Here's how the part is built. I have some questions about the finished solid (model axes, mm). Face numbers are marked on the shaded views. A direction names the side the tool comes from. Round coordinates to 2 decimals unless told otherwise and drop trailing zeros. Write each loop counter-clockwise with the first axis right and the second up, starting at its lowest first coordinate (ties: lowest second). Pieces come first, ordered by that corner, then holes. Notation, with made-up numbers: (82, 62) - (108, 62) arc R11 ccw to (108, 80) - close; hole circle Ø9 at (2.5, 53). An arc over 180 degrees is marked (long way). One line per question, with ' | ' between items. Start each with the question number.
(1) Imagine slicing it at A-A (y = 0). Write out the boundary of the cut face in (x, z), plus the area to 3 significant figures.
(2) Will these pins go through, and if not, where does the flat tip stop? pin 1 (4 mm diameter, centred on y = 8, z = 7.5, fed in from -X); pin 2 (12 mm diameter, centred on x = -42, y = 27.5, fed in from +Z); pin 3 (1 mm diameter, centred on y = -12.5, z = 2.5, fed in from +X).
(3) Thinking about a two-plate mould opening in X: for the marked faces 3, 4 and 5, which applies, pulls with the +X half, pulls with the -X half, needs draft (parallel to the pull), parting line crosses it, or undercut?
(4) For the marked faces 1 and 2, which set-ups out of +Z, -Z, +X, -X, +Y, -Y let a thin tool reach every point of the face, with its end or its side?
(5) If I drill on L1, parallel to X at y = 0, z = -9.5; L2, parallel to X at y = 0, z = 8, over which ranges is the centre line in solid material (lowest first)?
from build123d import *

# Parameters (mm, degrees)
F2_R    = 4
F3_R    = 2
F4_SIZE = 1


with BuildPart() as f1:
    # F0 (on Front) → F1 (revolve)
    with BuildSketch(Plane.XZ):
        Polygon((44.75, 18.25), (26.75, 18.25), (26.75, -18.25), (61.25, -18.25), (61.25, 7.38), (52, 7.38), (52, 13.95), (44.75, 13.95), align=None)
    revolve(axis=Axis((0, 0, -12.351525), (0, 0, -1)))

    # F2
    f2_edges = [f1.edges().sort_by_distance(p)[0] for p in [
        (-26.75, 0, 18.25),
        (-61.25, 0, -18.25),
    ]]
    fillet(f2_edges, radius=F2_R)

    # F3
    f3_edges = [f1.edges().sort_by_distance(p)[0] for p in [
        (-61.25, 0, 7.38),
    ]]
    fillet(f3_edges, radius=F3_R)

    # F4
    f4_edges = [f1.edges().sort_by_distance(p)[0] for p in [
        (-44.75, 0, 18.25),
        (-52, 0, 13.95),
        (-26.75, 0, -18.25),
    ]]
    chamfer(f4_edges, length=F4_SIZE)


solid = f1.part
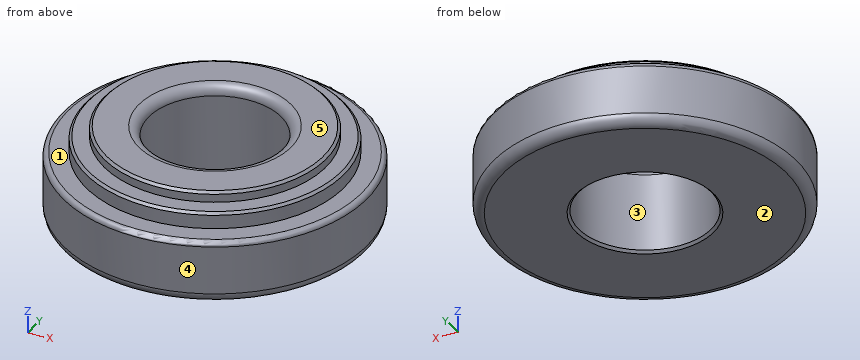
Check sheet entries:
1) outline: (-61.25, -14.25) arc R4 ccw to (-57.25, -18.25) - (-27.75, -18.25) - (-26.75, -17.25) - (-26.75, 14.25) arc R4 ccw to (-30.75, 18.25) - (-43.75, 18.25) - (-44.75, 17.25) - (-44.75, 13.95) - (-51, 13.95) - (-52, 12.95) - (-52, 7.38) - (-59.25, 7.38) arc R2 ccw to (-61.25, 5.38) - close; (26.75, -17.25) - (27.75, -18.25) - (57.25, -18.25) arc R4 ccw to (61.25, -14.25) - (61.25, 5.38) arc R2 ccw to (59.25, 7.38) - (52, 7.38) - (52, 12.95) - (51, 13.95) - (44.75, 13.95) - (44.75, 17.25) - (43.75, 18.25) - (30.75, 18.25) arc R4 ccw to (26.75, 14.25) - close | area: 2,240 mm^2
2) pin 1: x = -60.81 | pin 2: z = 17.8 | pin 3: x = 60.06
3) face 3: undercut | face 4: parting line crosses it | face 5: needs draft
4) face 1: +Z | face 2: -Z, +X, -X, +Y, -Y
5) L1: -61.25 to -26.75, 26.75 to 61.25 | L2: -52 to -26.75, 26.75 to 52
